Autodesk Inventor part; units mm, degrees
ref_plane "YZ Plane" through (0, 0, 0) normal (1, 0, 0) x (0, 1, 0)
ref_plane "XZ Plane" through (0, 0, 0) normal (0, 1, 0) x (-1, 0, 0)
ref_plane "XY Plane" through (0, 0, 0) normal (0, 0, 1) x (1, 0, 0)
sketch "Sketch1" plane through (0, 0, 0) normal (0, 0, 1) x (1, 0, 0)
  circle A0 centre (0, 0) radius 530
  dimension "d0" = 1060
extrude "Extrusion1" add sketch "Sketch1" along normal blind 200
sketch "Sketch2" plane through (0, 0, 200) normal (0, 0, 1) x (1, 0, 0)
  circle A0 centre (0, 0) radius 530
  line L0 (0, 0) -> (0, -300) construction
  line L1 (436.921, -300) -> (-436.921, -300)
  line L2 (-344.9012, -300) -> (-344.9012, 402.4216)
  line L3 (344.9012, -300) -> (344.9012, 402.4216)
  dimension "d3" = 300
  dimension "d5" = 873.8421
  dimension "d14" = 344.9012
extrude "Extrusion2" add sketch "Sketch2" along normal blind 250 contours L3 L1 L2 A0 | A0 L1
fillet "Fillet1" radius 100 1 edges at (0, -530, 450)
equation "\"d6\" = d9"
properties part number "02_DoF1_Podstawa"
Build history of the part. All positions in model axes, mm. A direction names the side the tool comes from. Give positions to 0.01 mm unless a question says otherwise; leave off trailing zeros. Loops run counter-clockwise (first coordinate to the right, second up) from the corner with the lowest first, then second, coordinate; pieces in that order, holes last. Notation, with made-up numbers: (-28.75, 86.25) - (-8.75, 86.25) arc R18 ccw to (-8.75, 120.25) - close; hole circle Ø7 at (52.5, -5). An arc over 180 degrees is marked (long way). Write item = value, one per line. Start each with the question number.
1) Band-saw the part on A-A on y = 0. Give the cut face in (x, z), plus the area to 3 significant figures.
2) Tool access for faces 1 (the flat face through (416, 56, 200)), 2 (the cylindrical face through (-114.894, 517.397, 171.85)), 3 (the flat face through (-390, -300, 321)): list every direction of +Z, -Z, +X, -X, +Y, -Y with a clear straight run to the whole face (end or side of a thin tool).
3) Probe probe 1 along X at (y, z) = (395.5, 334.5); probe 2 along Z at (x, y) = (386.5, -4); probe 3 along Y at (x, z) = (-179.5, 199). List the from-to ranges inside material, lowest first. Write a range as from..to.
4) Drop flat-ended pins along their axis: pin 1 Ø5 at (x, y) = (-354.5, -210) entering from +Z; pin 2 Ø8 at (y, z) = (-97.5, 102.5) entering from +X; pin 3 Ø6 at (y, z) = (251, 153) entering from +X. Give the stop position or say it passes through.
5) Band-saw the part on C-C on y = 188. Give the cut face in (x, z).
6) Band-saw the part on D-D on z = 231.5. Give the cut face in (x, y).
7) Band-saw the part on B-B on z = 155.5. Give the cut face in (x, y), plus the area to 3 significant figures.
Final values:
q1.outline = (-530, 0) - (530, 0) - (530, 200) - (344.9, 200) - (344.9, 450) - (-344.9, 450) - (-344.9, 200) - (-530, 200) - close
q1.area = 384,000 mm²
q2.face_1 = +Z, +X, +Y
q2.face_2 = +Z, -Z
q2.face_3 = +Z, -X, +Y
q3.probe_1 = -344.9..344.9
q3.probe_2 = 0..200
q3.probe_3 = -498.68..498.68
q4.pin_1 = 200
q4.pin_2 = 521.69
q4.pin_3 = 468.4
q5.outline = (-495.54, 0) - (495.54, 0) - (495.54, 200) - (344.9, 200) - (344.9, 450) - (-344.9, 450) - (-344.9, 200) - (-495.54, 200) - close
q6.outline = (-436.92, -300) arc R530 ccw to (436.92, -300) - (344.9, -300) - (344.9, 402.42) arc R530 ccw to (-344.9, 402.42) - (-344.9, -300) - close
q7.outline = circle Ø1060 at (0, 0)
q7.area = 882,000 mm²
